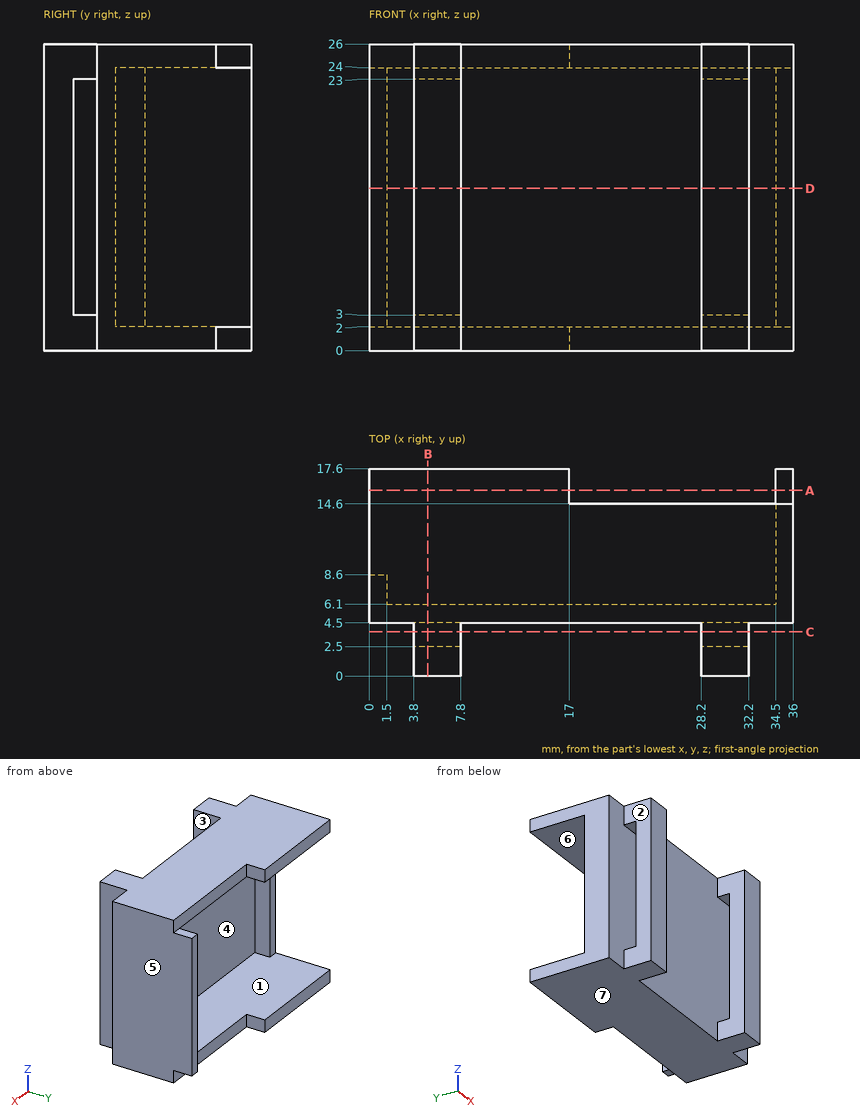
Part print with two shaded views. Sizes in mm from the minimum x, y, z corner. A direction names the side the tool comes from. Coordinates: 2 decimals unless noted, no trailing zeros. Order: outer loops, then holes, each group sorted by start corner. A loop starts at its lowest first (then second) coordinate and runs counter-clockwise, first axis right, second up. Notation, with made-up numbers: (21.5, 89) - (47.5, 89) arc R13 cw to (47.5, 113) - close; hole circle Ø8 at (75.25, 9). An arc over 180 degrees is marked (long way). Answer in a Markdown table with one row per item.
1. Slice it at D-D, the plane z = 13.75. List the corners of the cut face in (x, y).
Answer:
| item | result |
|---|---|
| outline | (0, 4.5) - (36, 4.5) - (36, 17.6) - (34.5, 17.6) - (34.5, 6.1) - (1.5, 6.1) - (1.5, 8.6) - (0, 8.6) - close; (3.8, 0) - (7.8, 0) - (7.8, 2.5) - (3.8, 2.5) - close; (28.2, 0) - (32.2, 0) - (32.2, 2.5) - (28.2, 2.5) - close |
2. 3-axis set-ups, long thin cutter, end or side, ignore diameter. For the marked faces 1, 2 and 3: which of +Z, -Z, +X, -X, +Y, -Y reach the whole face in a straight line?
Answer:
| item | result |
|---|---|
| face 1 | +Y |
| face 2 | +Z, -Z, -X, -Y |
| face 3 | +Z, -Z, -Y |
3. Slice it at C-C, the plane y = 3.75. List the corners of the cut face in (x, z).
Answer:
| item | result |
|---|---|
| outline | (3.8, 0) - (7.8, 0) - (7.8, 3) - (3.8, 3) - close; (3.8, 23) - (7.8, 23) - (7.8, 26) - (3.8, 26) - close; (28.2, 0) - (32.2, 0) - (32.2, 3) - (28.2, 3) - close; (28.2, 23) - (32.2, 23) - (32.2, 26) - (28.2, 26) - close |
4. Slice it at B-B, the plane x = 5. List the corners of the cut face in (y, z), then the cut area to 3 significant figures.
Answer:
| item | result |
|---|---|
| outline | (0, 0) - (17.6, 0) - (17.6, 2) - (6.1, 2) - (6.1, 24) - (17.6, 24) - (17.6, 26) - (0, 26) - close; hole (2.5, 3) - (4.5, 3) - (4.5, 23) - (2.5, 23) - close |
| area | 165 mm² |
5. Drill centre lines: L1, parallel to X at y = 6.75, z = 22.5; L2, parallel to Y at x = 6, z = 20.25; L3, parallel to Z at x = 31, y = 12. Where is each one in solid material? Low to high. Write a range as from..to.
Answer:
| item | result |
|---|---|
| L1 | 0..1.5, 34.5..36 |
| L2 | 0..2.5, 4.5..6.1 |
| L3 | 0..2, 24..26 |
6. Slice it at A-A, the plane y = 15.75. List the corners of the cut face in (x, z), then the cut area to 3 significant figures.
Answer:
| item | result |
|---|---|
| outline | (0, 0) - (17, 0) - (17, 2) - (0, 2) - close; (0, 24) - (17, 24) - (17, 26) - (0, 26) - close; (34.5, 2) - (36, 2) - (36, 24) - (34.5, 24) - close |
| area | 101 mm² |
7. Pull direction Z, two halves, no side cores. Call the marked faces 4, 5, 6 and 7: +Z half, -Z half, draft (parallel to the pull), parting line (faces both ways), or undercut.
Answer:
| item | result |
|---|---|
| face 4 | undercut |
| face 5 | draft |
| face 6 | undercut |
| face 7 | -Z half |
8. Flat gauge pins, fed straight in: P1, Ø0.6, axis at x = 27.5, z = 1, coming from the +Y side; P2, Ø4, axis at x = 27, y = 14.5, coming from the -Z side; P3, Ø0.8, axis at x = 35, y = 15.5, coming from the +Z side; P4, Ø10, axis at y = 14, z = 15.5, coming from the -X side. Where does each tip first touch, or does it go through?
Answer:
| item | result |
|---|---|
| P1 | y = 14.6 |
| P2 | z = 0 |
| P3 | z = 24 |
| P4 | x = 34.5 |
